```python
from build123d import *

# Parameters (mm, degrees)
SKETCH1_W             = 10
SKETCH1_H             = 10
SKETCH1_R             = 1.6
BOSS_EXTRUDE1_DEPTH   = 15
BOSS_EXTRUDE1_2_DEPTH = 15
BOSS_EXTRUDE2_DEPTH   = 10
FILLET1_R             = 15
FILLET2_R             = 3


with BuildPart() as part:
    # Sketch1 → Boss-Extrude1 (new body)
    with BuildSketch(Plane(origin=(0, 0, 0), x_dir=(1, 0, 0), z_dir=(0, 1, 0))):
        with Locations((-1.586813187, 40.5)):
            Rectangle(SKETCH1_W, SKETCH1_H)
        with Locations((-1.586813187, 40.5)):
            Circle(SKETCH1_R, mode=Mode.SUBTRACT)
    extrude(amount=BOSS_EXTRUDE1_DEPTH)



with BuildPart() as body_2:
    # Sketch1 → Boss-Extrude1 2 (new body)
    with BuildSketch(Plane(origin=(0, 0, 0), x_dir=(1, 0, 0), z_dir=(0, 1, 0))):
        with Locations((-1.586813187, -40.5)):
            Rectangle(SKETCH1_W, SKETCH1_H)
        with Locations((-1.586813187, -40.5)):
            Circle(SKETCH1_R, mode=Mode.SUBTRACT)
    extrude(amount=BOSS_EXTRUDE1_2_DEPTH)


with BuildPart() as part_1:
    add(part.part)

    add(body_2.part)  # Boss-Extrude2 merges body 2
    # Sketch4 → Boss-Extrude2 (add)
    with BuildSketch(Plane(origin=(3.413186813, 0, 0), x_dir=(0, 0, -1), z_dir=(1, 0, 0))):
        Polygon((-35.5, 15), (-24.25, 30), (24.25, 30), (35.5, 15), (45.5, 15), (28.25, 38), (-28.25, 38), (-45.5, 15), align=None)
    extrude(amount=-BOSS_EXTRUDE2_DEPTH)

    # Fillet1
    fillet1_edges = [part_1.edges().sort_by_distance(p)[0] for p in [
        (-1.586813187, 15, -35.5),
        (-1.586813187, 15, 35.5),
        (-1.586813187, 15, 45.5),
        (-1.586813187, 38, 28.25),
        (-1.586813187, 38, -28.25),
        (-1.586813187, 30, -24.25),
        (-1.586813187, 30, 24.25),
        (-1.586813187, 15, -45.5),
    ]]
    fillet(fillet1_edges, radius=FILLET1_R)

    # Fillet2
    fillet2_edges = [part_1.edges().sort_by_distance(p)[0] for p in [
        (-6.586813187, 5, 35.5),
        (3.413186813, 5, 35.5),
        (3.413186813, 21.5, 30.625),
        (-6.586813187, 21.5, 30.625),
        (3.413186813, 25.5, 37.625),
        (-6.586813187, 25.5, 37.625),
        (3.413186813, 5, -45.5),
        (3.413186813, 25.5, -37.625),
        (3.413186813, 38, 0),
        (3.413186813, 5, 45.5),
        (3.413186813, 30, 0),
        (3.413186813, 21.5, -30.625),
        (3.413186813, 5, -35.5),
        (3.413186813, 36.416407865, -27.458203932),
        (3.413186813, 14.74341649, -44.730249471),
        (3.413186813, 36.416407865, 27.458203932),
        (3.413186813, 14.74341649, 44.730249471),
        (-6.586813187, 5, 45.5),
        (-6.586813187, 5, -35.5),
        (-6.586813187, 21.5, -30.625),
        (-6.586813187, 30, 0),
        (-6.586813187, 38, 0),
        (-6.586813187, 25.5, -37.625),
        (-6.586813187, 5, -45.5),
        (-6.586813187, 36.416407865, -27.458203932),
        (-6.586813187, 14.74341649, -44.730249471),
        (-6.586813187, 36.416407865, 27.458203932),
        (-6.586813187, 14.74341649, 44.730249471),
        (3.413186813, 14.74341649, 34.730249471),
        (-6.586813187, 14.74341649, 34.730249471),
        (3.413186813, 28.416407865, 23.458203932),
        (-6.586813187, 28.416407865, 23.458203932),
        (3.413186813, 28.416407865, -23.458203932),
        (-6.586813187, 28.416407865, -23.458203932),
        (3.413186813, 14.74341649, -34.730249471),
        (-6.586813187, 14.74341649, -34.730249471),
    ]]
    fillet(fillet2_edges, radius=FILLET2_R)


solid = part_1.part
```
Design review of the part built by this model. Coordinates are the model's own, in mm. A direction names the side the tool comes from. Give positions to 0.01 mm unless a question says otherwise; leave off trailing zeros. Order: outer loops, then holes, each group sorted by start corner. A loop starts at its lowest first (then second) coordinate and runs counter-clockwise, first axis right, second up. Notation, with made-up numbers: M 89.25,-23 L 112.25,-23 A20 ccw 112.25,-9 Z; hole C 14.5,45.5 d2. An arc over 180 degrees is marked long. One line per question, with ' | ' between items. Start each with the question number.
Q1. We need section B-B (z = 14). Write out the cut boundary in (x, y), plus the area to 3 significant figures.
Q2. We need section C-C (x = -5.25). Write out the cut boundary in (y, z).
Q3. Machinability: for faces 4 (the face through (2.558, 5.07, 36.402)), 5 (the face through (-1.61, 36.46, 27.37)), 6 (the face through (-2, 5, 35.5)), which of the approach directions +Z, -Z, +X, -X, +Y, -Y give a long, thin tool a straight path to every point of the face, cutting with its end or side? Answer none if there is none.
Q4. The part is to be moulded in two halves that separate along Z. For faces 1 (the face through (-3, 0, 39)), 2 (the face through (2.56, 22.08, 31.32)), 3 (the face through (-5.73, 25.05, -36.84)), say which applies: +Z half, -Z half, draft (parallel to the pull), parting line (faces both ways), or undercut.
Q5. For L1, parallel to Z at x = -0.5, y = 12; L2, parallel to X at y = 10.5, z = 40.5; L3, parallel to Z at x = -5.5, y = 5.5, list the stretches that pass through material, from the lowest coordinate up. Write a range as [from, to].
Q6. We need section A-A (y = 3). Write out the cut boundary in (x, z), plus the area to 3 significant figures.
Q7. For pin 1 Ø2 at (x, z) = (-5, -10) entering from +Y; pin 2 Ø1.9 at (x, z) = (-1.59, 40.5) entering from -Y; pin 3 Ø5 at (x, z) = (-1.59, -40.5) entering from +Y, all flat-tipped, find the tip position at first contact; note any pin that passes through.
Q8. We need section D-D (y = 13.5). State how many separate pieces and enclosed holes the cut face has, plus the area to 3 significant figures.
Returned:
1) outline: M -6.59,33 A3 ccw -3.59,30 L 0.41,30 A3 ccw 3.41,33 L 3.41,35 A3 ccw 0.41,38 L -3.59,38 A3 ccw -6.59,35 Z | area: 72.3 mm2
2) outline: M 0,-45 L 10,-45 A14.5 ccw 18.7,-42.1 L 31.7,-32.35 A14.5 ccw 37.5,-20.75 L 37.5,20.75 A14.5 ccw 31.7,32.35 L 18.7,42.1 A14.5 ccw 10,45 L 0,45 L 0,36 L 10,36 A15.5 cw 19.3,32.9 L 24.3,29.15 A15.5 cw 30.5,16.75 L 30.5,-16.75 A15.5 cw 24.3,-29.15 L 19.3,-32.9 A15.5 cw 10,-36 L 0,-36 Z
3) face 4: +X, -Y | face 5: +Z, +X, -X, +Y | face 6: +X, -X, -Y
4) face 1: draft | face 2: undercut | face 3: -Z half
5) L1: [-45.37, -41.67], [-39.33, -35.37], [35.37, 39.33], [41.67, 45.37] | L2: [-6.59, -3.19], [0.01, 3.41] | L3: [-44.81, -36.19], [36.19, 44.81]
6) outline: M -6.59,-42.5 A3 ccw -3.59,-45.5 L 0.41,-45.5 A3 ccw 3.41,-42.5 L 3.41,-38.5 A3 ccw 0.41,-35.5 L -3.59,-35.5 A3 ccw -6.59,-38.5 Z; M -6.59,38.5 A3 ccw -3.59,35.5 L 0.41,35.5 A3 ccw 3.41,38.5 L 3.41,42.5 A3 ccw 0.41,45.5 L -3.59,45.5 A3 ccw -6.59,42.5 Z; hole C -1.59,-40.5 d3.2; hole C -1.59,40.5 d3.2 | area: 168 mm2
7) pin 1: y = 37.97 | pin 2: y = 15 | pin 3: y = 25
8) separate pieces: 2 | enclosed holes: 2 | area: 168 mm2
